For this review, take the finished solid that the model builds, in its own axes (mm). A direction names the side the tool comes from. Coordinates: 2 decimals unless noted, no trailing zeros. Loops run counter-clockwise (first coordinate to the right, second up) from the corner with the lowest first, then second, coordinate; pieces in that order, holes last. Notation, with made-up numbers: M -35.75,29.25 L 20.25,29.25 A11 cw 20.25,35.25 Z; hole C -25,41 d1. An arc over 180 degrees is marked long. Put each result on its own line as item: value.
```python
from build123d import *

# Parameters (mm, degrees)
PAD_DEPTH          = 55
SKETCH001_W        = 72
SKETCH001_H        = 51
POCKET_DEPTH       = 30
SKETCH002_W        = 30
SKETCH002_H        = 89
PAD001_DEPTH       = 51
PAD001_FACE5_W     = 30
PAD001_FACE5_H     = 60
PAD002_DEPTH       = 1
PAD002_FACE31_W    = 30
PAD002_FACE31_H    = 60
PAD003_DEPTH       = 1
SKETCH003_W        = 87
SKETCH003_H        = 51
POCKET001_DEPTH    = 27
SKETCH004_W        = 71
SKETCH004_H        = 51
POCKET002_DEPTH    = 2
SKETCH005_W        = 62
SKETCH005_H        = 47
POCKET003_DEPTH    = 1
SKETCH006_R        = 1.5
PAD004_DEPTH       = 2
POCKET004_DEPTH    = 55.001
SKETCH008_W        = 30
SKETCH008_H        = 51
POCKET005_DEPTH    = 2
POCKET005_FACE21_W = 51
POCKET005_FACE21_H = 1
POCKET006_DEPTH    = 2
POCKET007_DEPTH    = 88


with BuildPart() as part:
    # Sketch → Pad (new body)
    with BuildSketch(Plane.YZ):
        with BuildLine():
            Line((0, 0), (-30, 0))
            Line((-30, 0), (-30, 3))
            Line((-30, 3), (-67, 3))
            ThreePointArc((-67, 9), (-70, 6), (-67, 3))
            Line((-67, 9), (-52, 9))
            Line((-52, 9), (-52, 17))
            ThreePointArc((-72, 32), (-64.630858, 20.992189), (-52, 17))
            Line((-72, 32), (0, 32))
            Line((0, 32), (0, 0))
        make_face()
    extrude(amount=PAD_DEPTH)

    # Sketch001 (on Face1 of Pad) → Pocket (cut)
    with BuildSketch(Plane(origin=(0, 0, 32), x_dir=(0, -1, 0), z_dir=(0, 0, 1))):
        with Locations((36, 27.5)):
            Rectangle(SKETCH001_W, SKETCH001_H)
    extrude(amount=-POCKET_DEPTH, mode=Mode.SUBTRACT)

    # Sketch002 (on Face14 of Pocket) → Pad001 (join)
    with BuildSketch(Plane(origin=(53, 0, 0), x_dir=(0, 1, 0), z_dir=(-1, 0, 0))):
        with Locations((-37, -47.5)):
            Rectangle(SKETCH002_W, SKETCH002_H)
    extrude(amount=PAD001_DEPTH)

    # Pad001 Face5 → Pad002 (add)
    with BuildSketch(Plane(origin=(2, -37, 62), x_dir=(0, 1, 0), z_dir=(-1, 0, 0))):
        Rectangle(PAD001_FACE5_W, PAD001_FACE5_H)
    extrude(amount=PAD002_DEPTH)

    # Pad002 Face31 → Pad003 (add)
    with BuildSketch(Plane(origin=(53, -37, 62), x_dir=(0, -1, 0), z_dir=(1, 0, 0))):
        Rectangle(PAD002_FACE31_W, PAD002_FACE31_H)
    extrude(amount=PAD003_DEPTH)

    # Sketch003 (on Face23 of Pad003) → Pocket001 (cut)
    with BuildSketch(Plane(origin=(0, -52, 0), x_dir=(0, 0, -1), z_dir=(0, -1, 0))):
        with Locations((-47.5, 27.5)):
            Rectangle(SKETCH003_W, SKETCH003_H)
    extrude(amount=-POCKET001_DEPTH, mode=Mode.SUBTRACT)

    # Sketch004 (on Face39 of Pocket001) → Pocket002 (cut)
    with BuildSketch(Plane(origin=(0, -25, 0), x_dir=(0, 0, -1), z_dir=(0, -1, 0))):
        with Locations((-49.5, 27.5)):
            Rectangle(SKETCH004_W, SKETCH004_H)
    extrude(amount=-POCKET002_DEPTH, mode=Mode.SUBTRACT)

    # Sketch005 (on Face47 of Pocket002) → Pocket003 (cut)
    with BuildSketch(Plane(origin=(0, -23, 0), x_dir=(0, 0, -1), z_dir=(0, -1, 0))):
        with Locations((-51, 27.5)):
            Rectangle(SKETCH005_W, SKETCH005_H)
    extrude(amount=-POCKET003_DEPTH, mode=Mode.SUBTRACT)

    # Sketch006 (on Face43 of Pocket003) → Pad004 (join)
    with BuildSketch(Plane(origin=(0, -25, 0), x_dir=(0, 0, -1), z_dir=(0, -1, 0))):
        with BuildLine():
            Line((-8.5, 2), (-14, 2))
            Line((-14, 2), (-14, 7.158312))
            ThreePointArc((-8.5, 5.5), (-10.633975, 8.372281), (-14, 7.158312))
            Line((-8.5, 2), (-8.5, 5.5))
        make_face()
        with Locations((-11.5, 5.5)):
            Circle(SKETCH006_R, mode=Mode.SUBTRACT)
        with BuildLine():
            Line((-14, 47.841688), (-14, 53))
            Line((-14, 53), (-8.5, 53))
            Line((-8.5, 53), (-8.5, 49.5))
            ThreePointArc((-14, 47.841688), (-10.633975, 46.627719), (-8.5, 49.5))
        make_face()
        with Locations((-11.5, 49.5)):
            Circle(SKETCH006_R, mode=Mode.SUBTRACT)
        with BuildLine():
            Line((-85, 7.158312), (-85, 2))
            Line((-85, 2), (-91, 2))
            Line((-91, 2), (-91, 8.5))
            Line((-91, 8.5), (-87.5, 8.5))
            ThreePointArc((-85, 7.158312), (-86.081363, 8.143382), (-87.5, 8.5))
        make_face()
        with Locations((-87.5, 5.5)):
            Circle(SKETCH006_R, mode=Mode.SUBTRACT)
        with BuildLine():
            Line((-85, 47.841688), (-85, 53))
            Line((-85, 53), (-91, 53))
            Line((-91, 53), (-91, 46.5))
            Line((-91, 46.5), (-87.5, 46.5))
            ThreePointArc((-87.5, 46.5), (-86.081363, 46.856618), (-85, 47.841688))
        make_face()
        with Locations((-87.5, 49.5)):
            Circle(SKETCH006_R, mode=Mode.SUBTRACT)
    extrude(amount=PAD004_DEPTH)

    # Sketch007 (on Face16 of Pad004) → Pocket004 (cut, through all)
    with BuildSketch(Plane.YZ.offset(55)):
        Polygon((0.114911, 10), (0.114911, 32), (-21.885089, 32), align=None)
    extrude(amount=-POCKET004_DEPTH, mode=Mode.SUBTRACT)

    # Sketch008 (on Face15 of Pocket004) → Pocket005 (cut)
    with BuildSketch(Plane.YX):
        with Locations((-15, 27.5)):
            Rectangle(SKETCH008_W, SKETCH008_H)
    extrude(amount=-POCKET005_DEPTH, mode=Mode.SUBTRACT)

    # Pocket005 Face21 → Pocket006 (cut)
    with BuildSketch(Plane(origin=(27.5, -52, 91.5), x_dir=(-1, 0, 0), z_dir=(0, -1, 0))):
        Rectangle(POCKET005_FACE21_W, POCKET005_FACE21_H)
    extrude(amount=-POCKET006_DEPTH, mode=Mode.SUBTRACT)

    # Sketch009 (on Face20 of Pocket006) → Pocket007 (cut)
    with BuildSketch(Plane(origin=(0, 0, 92), x_dir=(0, -1, 0), z_dir=(0, 0, 1))):
        Polygon((52, 53), (50, 53), (50, 53.6), align=None)
        Polygon((52, 2), (50, 2), (50, 1.4), align=None)
    extrude(amount=-POCKET007_DEPTH, mode=Mode.SUBTRACT)


solid = part.part
```
(1) Wall thickness on line 1 along X through (y, z) = (-25.85, 87.5); line 2 along X through (y, z) = (-53.5, 7); line 3 along X through (y, z) = (-26, 87): over which ranges is each line inside the solid? List them lowest first. Write a range as [from, to].
Determined:
line 1: x = [1, 4], [7, 8.5], [46.5, 48], [51, 54]
line 2: x = [0, 2], [53, 55]
line 3: x = [1, 4.09], [6.91, 8.46], [46.54, 48.09], [50.91, 54]
(2) Add section D-D (y = -39). Write out the cut boundary in (x, z), plus the area to 3 significant figures.
Determined:
outline: M 0,3 L 55,3 L 55,32 L 54,32 L 54,92 L 1,92 L 1,32 L 0,32 Z; hole M 2,4 L 53,4 L 53,91 L 2,91 Z
area: 338 mm^2
(3) Add section A-A (x = 45). Write out the cut boundary in (y, z).
Determined:
outline: M -52,3 L -22,3 L -22,20 L -23,20 L -23,14 L -25,14 L -25,4 L -52,4 Z; M -50,91 L -25,91 L -25,85 L -23,85 L -23,82 L -22,82 L -22,92 L -50,92 Z
(4) Add section B-B (z = 45). Write out the cut boundary in (x, y).
Determined:
outline: M 1,-52 L 2,-52 L 1.4,-50 L 2,-50 L 2,-23 L 4,-23 L 4,-22 L 1,-22 Z; M 51,-23 L 53,-23 L 53,-50 L 53.6,-50 L 53,-52 L 54,-52 L 54,-22 L 51,-22 Z
(5) Draft analysis for pull direction X (two halves, no side actions). For faces 1 (the flat face through (0, -35, 16)), 2 (the flat face through (8.5, -26, 89)), 3 (the flat face through (1, -15, 0)), 4 (the flat face through (2, -36, 48)), state which applies: +X half, -X half, draft (parallel to the pull), parting line (faces both ways), or undercut.
Determined:
face 1: -X half
face 2: undercut
face 3: draft
face 4: undercut
(6) Tool access review of faces 5 (the flat face through (53, -61, 6)), 6 (the flat face through (51, -27, 89)), 7 (the flat face through (54, -30, 1)): name each direction out of +Z, -Z, +X, -X, +Y, -Y from which nothing blocks a thin tool from reaching the whole face with its end or side.
Determined:
face 5: +Z, -Z, -Y
face 6: -Y
face 7: -Z, +X, -X, -Y
(7) Add section C-C (y = -9). Write out the cut boundary in (x, z), plus the area to 3 significant figures.
Determined:
outline: M 0,0 L 2,0 L 2,19.11 L 0,19.11 Z; M 53,0 L 55,0 L 55,19.11 L 53,19.11 Z
area: 76.5 mm^2
(8) For pin 1 (1.5 mm diameter, centred on y = -51.5, z = 69.5, fed in from -X); pin 2 (0.6 mm diameter, centred on y = -25.5, z = 90, fed in from +X); pin 3 (1.7 mm diameter, centred on x = 49, z = 10, fed in from -Y); pin 4 (6 mm diameter, centred on x = 34.5, z = 78, fed in from +Y), all flat-tipped, find the tip position at first contact; note any pin that passes through.
Determined:
pin 1: stops at x = 1
pin 2: stops at x = 54
pin 3: stops at y = -27
pin 4: passes through
